Part model, mm, in its own coordinate system. A direction names the side the tool comes from. Round coordinates to 2 decimals unless told otherwise and drop trailing zeros. Order: outer loops, then holes, each group sorted by start corner. A loop starts at its lowest first (then second) coordinate and runs counter-clockwise, first axis right, second up. Notation, with made-up numbers: (36.5, -36.75) -> (65.5, -36.75) arc R20 ccw to (65.5, -23.75) -> close; hole circle Ø3 at (81, 60.25). An arc over 180 degrees is marked (long way). Use CSV: the item, a comma, the result in double quotes.
```python
from build123d import *

# Parameters (mm, degrees)
SKETCH1_W           = 80
SKETCH1_H           = 6
BOSS_EXTRUDE1_DEPTH = 50
SKETCH6_R           = 20
BOSS_EXTRUDE2_DEPTH = 15
BOSS_EXTRUDE3_START = 25
SKETCH7_R           = 20
BOSS_EXTRUDE3_DEPTH = 25
CUT_EXTRUDE1_REACH  = 90.639
SKETCH8_R           = 10
CUT_EXTRUDE2_REACH  = 79.342
SKETCH9_R           = 5


with BuildPart() as part:
    # Sketch1 → Boss-Extrude1 (new body)
    with BuildSketch(Plane.XY):
        with Locations((1.914357683, -3)):
            Rectangle(SKETCH1_W, SKETCH1_H)
    extrude(amount=-BOSS_EXTRUDE1_DEPTH)


with BuildPart() as part_1:
    # Body-Move/Copy2: moved
    add(part.part.moved(Location((0, 0, 25))))

    # Sketch6 → Boss-Extrude2 (add)
    with BuildSketch(Plane.XY):
        with BuildLine():
            Line((-38.085642317, 0), (41.914357683, 0))
            Line((41.914357683, 0), (26.914357683, 40))
            Line((26.914357683, 40), (21.914357683, 40))
            ThreePointArc((21.914357683, 40), (1.914357683, 20), (-18.085642317, 40))
            Line((-18.085642317, 40), (-23.085642317, 40))
            Line((-23.085642317, 40), (-38.085642317, 0))
        make_face()
        with Locations((1.914357683, 40)):
            Circle(SKETCH6_R)
    extrude(amount=-BOSS_EXTRUDE2_DEPTH)

    # Sketch7 → Boss-Extrude3 (add)
    with BuildSketch(Plane.XY.offset(BOSS_EXTRUDE3_START)):
        with Locations((1.914357683, 40)):
            Circle(SKETCH7_R)
    extrude(amount=-BOSS_EXTRUDE3_DEPTH)

    # Sketch8 → Cut-Extrude1 (cut, up to next)
    with BuildSketch(Plane.XY.offset(25), mode=Mode.PRIVATE) as cut_extrude1_sk1:
        with Locations((1.914357683, 40)):
            Circle(SKETCH8_R)
    cut_extrude1_tool1 = extrude(cut_extrude1_sk1.sketch, amount=-CUT_EXTRUDE1_REACH, mode=Mode.PRIVATE) & part_1.part
    add(cut_extrude1_tool1.solids().sort_by_distance((1.914358, 40, 25))[0], mode=Mode.SUBTRACT)

    # Sketch9 → Cut-Extrude2 (cut, up to next)
    with BuildSketch(Plane(origin=(0, 0, 0), x_dir=(1, 0, 0), z_dir=(0, 1, 0)), mode=Mode.PRIVATE) as cut_extrude2_sk1:
        with Locations(Location((26.914357683, -12, 0), (0, 0, 270))):
            Circle(SKETCH9_R)
    cut_extrude2_tool1 = extrude(cut_extrude2_sk1.sketch, amount=-CUT_EXTRUDE2_REACH, mode=Mode.PRIVATE) & part_1.part
    # Sketch9 → Cut-Extrude2 (cut, up to next)
    with BuildSketch(Plane(origin=(0, 0, 0), x_dir=(1, 0, 0), z_dir=(0, 1, 0)), mode=Mode.PRIVATE) as cut_extrude2_sk2:
        with Locations(Location((-23.085642317, -12, 0), (0, 0, 270))):
            Circle(SKETCH9_R)
    cut_extrude2_tool2 = extrude(cut_extrude2_sk2.sketch, amount=-CUT_EXTRUDE2_REACH, mode=Mode.PRIVATE) & part_1.part
    add(cut_extrude2_tool1.solids().sort_by_distance((26.914358, 0, 12))[0], mode=Mode.SUBTRACT)
    add(cut_extrude2_tool2.solids().sort_by_distance((-23.085642, 0, 12))[0], mode=Mode.SUBTRACT)


solid = part_1.part
```
(1) Drop flat-ended pins along their axis: P1, Ø1, axis at x = 12, y = 13.5, coming from the -Z side; P2, Ø1, axis at x = 1, z = 15, coming from the +Y side; P3, Ø1, axis at y = 33.5, z = 7, coming from the +X side; P4, Ø16, axis at x = 1.91, y = 40, coming from the -Z side. Give the stop position or say it passes through.
Reply:
P1,"z = -15"
P2,"y = 60"
P3,"x = 20.99"
P4,"through"
(2) Probe probe 1 along X at (y, z) = (-4, 12); probe 2 along Y at (x, z) = (9, 1); probe 3 along Y at (x, z) = (-2.5, 13). List the from-to ranges inside material, lowest first. Write a range as [from, to].
Reply:
probe 1,"[-38.09, -28.09], [-18.09, 21.91], [31.91, 41.91]"
probe 2,"[-6, 0], [21.3, 32.94], [47.06, 58.7]"
probe 3,"[-6, 0], [20.49, 31.03], [48.97, 59.51]"
(3) Cut at A-A, the plane z = 1.5. Give the cut face in (x, y), then the cut area to 3 significant figures.
Reply:
outline,"(-38.09, -6) -> (41.91, -6) -> (41.91, 0) -> (-38.09, 0) -> close; circle Ø40 at (1.91, 40); hole circle Ø20 at (1.91, 40)"
area,"1,420 mm2"
(4) Which spindle directions (+Z, -Z, +X, -X, +Y, -Y) get a long thin tool onto all of the face, cutting with end or side? Do faces 5 (the face through (1, 16, 0)), 6 (the face through (1, 24, -15)), 7 (the face through (1, 0, 13)), 8 (the face through (24, 40, -7)), 9 (the face through (-21, 40, -7)). Say none if no direction does.
Reply:
face 5,"+Z"
face 6,"-Z, +X, -X, +Y"
face 7,"+Z, +X, -X"
face 8,"+Z, -Z, +X, +Y"
face 9,"+Z, -Z, -X, +Y"
(5) Cut at D-D, the plane y = 21. Give the cut face in (x, z).
Reply:
outline,"(-30.21, -15) -> (34.04, -15) -> (34.04, 0) -> (8.16, 0) -> (8.16, 25) -> (-4.33, 25) -> (-4.33, 0) -> (-30.21, 0) -> close"
(6) Cut at C-C, the plane x = 5.5. Give the cut face in (y, z).
Reply:
outline,"(-6, -25) -> (0, -25) -> (0, -15) -> (30.66, -15) -> (30.66, 25) -> (20.32, 25) -> (20.32, 0) -> (0, 0) -> (0, 25) -> (-6, 25) -> close; (49.34, -15) -> (59.68, -15) -> (59.68, 25) -> (49.34, 25) -> close"
(7) Cut at B-B, the plane z = 12. Give the cut face in (x, y).
Reply:
outline,"(-38.09, -6) -> (-28.09, -6) -> (-28.09, 0) -> (-38.09, 0) -> close; (-18.09, -6) -> (21.91, -6) -> (21.91, 0) -> (-18.09, 0) -> close; circle Ø40 at (1.91, 40); (31.91, -6) -> (41.91, -6) -> (41.91, 0) -> (31.91, 0) -> close; hole circle Ø20 at (1.91, 40)"
(8) Pull direction X, two halves, no side cores. Call faces 1 (the face through (-0.253, 30.238, 5.28)), 2 (the face through (1, 0, -20)), 3 (the face through (28.42, -2.96, 16.77)), 4 (the face through (-38.086, -3, 0)): released by +X, released by -X, zero draft, split by the parting line, or undercut.
Reply:
face 1,"undercut"
face 2,"zero draft"
face 3,"undercut"
face 4,"released by -X"
